from build123d import *

# Parameters (mm, degrees)
SKETCH1_W           = 154.94
SKETCH1_H           = 154.94
BOSS_EXTRUDE1_DEPTH = 15.24
SKETCH3_W           = 15.24
SKETCH3_H           = 30.988
SKETCH3_W_2         = 30.988
SKETCH3_H_2         = 15.24
CUT_EXTRUDE1_DEPTH  = 220.647592293
CUT_EXTRUDE2_DEPTH  = 220.647592293


with BuildPart() as part:
    # Sketch1 → Boss-Extrude1 (new body)
    with BuildSketch(Plane.XY):
        with Locations((77.47, 77.47)):
            Rectangle(SKETCH1_W, SKETCH1_H)
    extrude(amount=BOSS_EXTRUDE1_DEPTH)

    # Sketch3 → Cut-Extrude1 (cut, through all)
    with BuildSketch(Plane.XY.offset(15.24)):
        with Locations((7.62, 108.458)):
            Rectangle(SKETCH3_W, SKETCH3_H)
        with Locations((7.62, 46.482)):
            Rectangle(SKETCH3_W, SKETCH3_H)
        with Locations((147.32, 108.458)):
            Rectangle(SKETCH3_W, SKETCH3_H)
        with Locations((147.32, 46.482)):
            Rectangle(SKETCH3_W, SKETCH3_H)
        with Locations((46.482, 147.32)):
            Rectangle(SKETCH3_W_2, SKETCH3_H_2)
        with Locations((108.458, 147.32)):
            Rectangle(SKETCH3_W_2, SKETCH3_H_2)
        with Locations((46.482, 7.62)):
            Rectangle(SKETCH3_W_2, SKETCH3_H_2)
        with Locations((108.458, 7.62)):
            Rectangle(SKETCH3_W_2, SKETCH3_H_2)
    extrude(amount=-CUT_EXTRUDE1_DEPTH, mode=Mode.SUBTRACT)

    # Sketch7 → Cut-Extrude2 (cut, through all)
    with BuildSketch(Plane.XY.offset(15.24)):
        with BuildLine():
            Line((21.47466448, 66.04), (24.069558054, 66.04))
            ThreePointArc((24.069558054, 66.04), (22.86, 77.47), (24.069558054, 88.9))
            Line((24.069558054, 88.9), (21.47466448, 88.9))
            ThreePointArc((21.47466448, 88.9), (20.32, 77.47), (21.47466448, 66.04))
        make_face()
        with BuildLine():
            Line((88.9, 24.069558054), (88.9, 21.47466448))
            ThreePointArc((88.9, 21.47466448), (77.47, 20.32), (66.04, 21.47466448))
            Line((66.04, 21.47466448), (66.04, 24.069558054))
            ThreePointArc((66.04, 24.069558054), (77.47, 22.86), (88.9, 24.069558054))
        make_face()
        with BuildLine():
            Line((130.870441946, 88.9), (133.46533552, 88.9))
            ThreePointArc((133.46533552, 88.9), (134.62, 77.47), (133.46533552, 66.04))
            Line((133.46533552, 66.04), (130.870441946, 66.04))
            ThreePointArc((130.870441946, 66.04), (132.08, 77.47), (130.870441946, 88.9))
        make_face()
        with BuildLine():
            Line((88.9, 133.46533552), (88.9, 130.870441946))
            ThreePointArc((88.9, 130.870441946), (77.47, 132.08), (66.04, 130.870441946))
            Line((66.04, 130.870441946), (66.04, 133.46533552))
            ThreePointArc((66.04, 133.46533552), (77.47, 134.62), (88.9, 133.46533552))
        make_face()
    extrude(amount=-CUT_EXTRUDE2_DEPTH, mode=Mode.SUBTRACT)


solid = part.part
Could you check a few things on this model? Use its own coordinates, in mm. A direction names the side the tool comes from. Coordinates: 2 decimals unless noted, no trailing zeros. Loops run counter-clockwise (first coordinate to the right, second up) from the corner with the lowest first, then second, coordinate; pieces in that order, holes last.
1. Imagine slicing it at A-A (y = 12.5). Please give me the cut outline in (x, z), and give its area (3 significant figures).
2. Imagine slicing it at D-D (x = 103.5). Please give me the cut outline in (y, z).
3. I need wall thicknesses on L1, parallel to X at y = 7, z = 8; L2, parallel to X at y = 77.5, z = 9.75. Which ranges of each line are inside material? Lowest first, please.
4. Imagine slicing it at C-C (y = 70). Please give me the cut outline in (x, z), and give its area (3 significant figures).
5. For faces 4 (the face through (147, 61.976, 8)), 5 (the face through (134.62, 77.63, 7.73)), 6 (the face through (30.988, 8, 8)), 7 (the face through (8, 92.964, 8)), which set-ups out of +Z, -Z, +X, -X, +Y, -Y let a thin tool reach every point of the face, with its end or its side?
6. Imagine slicing it at B-B (z = 9.5). Give the number of separate pieces and of enclosed holes in the cut face, and give its area (3 significant figures).
7. We'd pull the mould along Y, two halves only. Please class faces 1 (the face through (76, 79, 15.24)), 2 (the face through (15.24, 46, 8)), 3 (the face through (15, 154.94, 8)): released by +Y, released by -Y, zero draft, split by the parting line, or undercut.
8. For P1, Ø7.5, axis at y = 40, z = 8, coming from the -X side; P2, Ø7.5, axis at x = 47, z = 11, coming from the -Y side; P3, Ø4.5, axis at y = 43, z = 10.5, coming from the +X side, each with a flat end and sliding along its axis, tell me the tip position at first contact or that it passes through.
Computed values:
1. outline: (0, 0) - (30.99, 0) - (30.99, 15.24) - (0, 15.24) - close; (61.98, 0) - (92.96, 0) - (92.96, 15.24) - (61.98, 15.24) - close; (123.95, 0) - (154.94, 0) - (154.94, 15.24) - (123.95, 15.24) - close
1. area: 1,420 mm2
2. outline: (15.24, 0) - (139.7, 0) - (139.7, 15.24) - (15.24, 15.24) - close
3. L1: x = 0 to 30.99, 61.98 to 92.96, 123.95 to 154.94
3. L2: x = 0 to 20.32, 22.86 to 132.08, 134.62 to 154.94
4. outline: (0, 0) - (20.81, 0) - (20.81, 15.24) - (0, 15.24) - close; (23.37, 0) - (131.57, 0) - (131.57, 15.24) - (23.37, 15.24) - close; (134.13, 0) - (154.94, 0) - (154.94, 15.24) - (134.13, 15.24) - close
4. area: 2,280 mm2
5. face 4: +Z, -Z, +X
5. face 5: +Z, -Z
5. face 6: +Z, -Z, -Y
5. face 7: +Z, -Z, -X
6. separate pieces: 1
6. enclosed holes: 4
6. area: 20,000 mm2
7. face 1: zero draft
7. face 2: undercut
7. face 3: released by +Y
8. P1: stops at x = 15.24
8. P2: stops at y = 15.24
8. P3: stops at x = 139.7
